Part model, mm, in its own coordinate system. Round coordinates to 2 decimals unless told otherwise and drop trailing zeros. Loops run counter-clockwise (first coordinate to the right, second up) from the corner with the lowest first, then second, coordinate; pieces in that order, holes last. Notation, with made-up numbers: M -31,42.25 L 3,42.25 A25 cw 3,64.25 Z; hole C -6.75,-31 d8. An arc over 180 degrees is marked long. Answer as CSV lines item,"result". Start each with the question number.
Item 1: Band-saw the part on B-B (x = 311.5). Give the cut face in (y, z), and give its area (3 significant figures).
Item 2: Wall check: line 1 (X direction, y = 6, z = 0.1); line 2 (Y direction, x = 303, z = 2.75); line 3 (X direction, y = 19.5, z = 2.5). Give the ranges that are in metal, low to high.
Item 3: Band-saw the part on C-C (x = 125.25). Give the cut face in (y, z), and give its area (3 significant figures).
Item 4: Drop flat-ended pins along their axis: pin 1 Ø1 at (x, y) = (124.5, 62.5) entering from -Z; pin 2 Ø1.5 at (y, z) = (8, 1) entering from +X; pin 3 Ø1.5 at (x, z) = (284, 2) entering from -Y; pin 4 Ø1 at (y, z) = (25, 0.5) entering from +X. Give the stop position or say it passes through.
Item 5: Band-saw the part on A-A (y = 8). Give the cut face in (x, z), and give its area (3 significant figures).
```python
from build123d import *

# Parameters (mm, degrees)
PAD_DEPTH = 3


with BuildPart() as part:
    # Sketch → Pad (new body)
    with BuildSketch(Plane.XY):
        with BuildLine():
            Line((0, 100.6), (0, 1))
            ThreePointArc((0, 1), (0.292893, 0.292893), (1, 0))
            Line((1, 0), (14.748, 0))
            ThreePointArc((14.748, 0), (15.455107, 0.292893), (15.748, 1))
            Line((15.748, 12.7), (15.748, 1))
            ThreePointArc((22.352, 12.7), (19.05, 16.002), (15.748, 12.7))
            Line((22.352, 12.7), (22.352, 1))
            ThreePointArc((22.352, 1), (22.644893, 0.292893), (23.352, 0))
            Line((23.352, 0), (120.948, 0))
            ThreePointArc((120.948, 0), (121.655107, 0.292893), (121.948, 1))
            Line((121.948, 12.7), (121.948, 1))
            ThreePointArc((128.552, 12.7), (125.25, 16.002), (121.948, 12.7))
            Line((128.552, 12.7), (128.552, 1))
            ThreePointArc((128.552, 1), (128.844893, 0.292893), (129.552, 0))
            Line((129.552, 0), (227.148, 0))
            ThreePointArc((227.148, 0), (227.855107, 0.292893), (228.148, 1))
            Line((228.148, 12.7), (228.148, 1))
            ThreePointArc((234.752, 12.7), (231.45, 16.002), (228.148, 12.7))
            Line((234.752, 12.7), (234.752, 1))
            ThreePointArc((234.752, 1), (235.044893, 0.292893), (235.752, 0))
            Line((235.752, 0), (249.5, 0))
            ThreePointArc((249.5, 0), (250.207107, 0.292893), (250.5, 1))
            Line((250.5, 1), (250.5, 24.9))
            ThreePointArc((251.5, 25.9), (250.792893, 25.607107), (250.5, 24.9))
            Line((251.5, 25.9), (330.9999, 25.9))
            ThreePointArc((330.9999, 25.9), (331.707007, 26.192893), (331.9999, 26.9))
            Line((331.9999, 26.9), (331.9999, 100.6))
            ThreePointArc((331.9999, 100.6), (331.707007, 101.307107), (330.9999, 101.6))
            Line((330.9999, 101.6), (1, 101.6))
            ThreePointArc((1, 101.6), (0.292893, 101.307107), (0, 100.6))
        make_face()
    extrude(amount=PAD_DEPTH)


solid = part.part
```
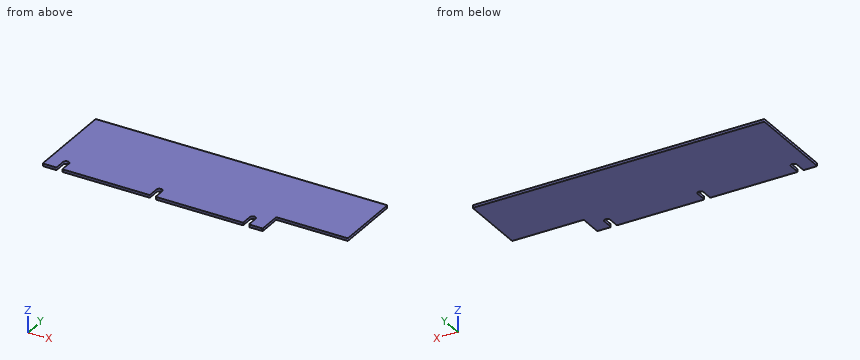
Answer block:
1,outline,"M 25.9,0 L 101.6,0 L 101.6,3 L 25.9,3 Z"
1,area,"227 mm^2"
2,line 1,"x = 0 to 15.75, 22.35 to 121.95, 128.55 to 228.15, 234.75 to 250.5"
2,line 2,"y = 25.9 to 101.6"
2,line 3,"x = 0 to 250.5"
3,outline,"M 16,0 L 101.6,0 L 101.6,3 L 16,3 Z"
3,area,"257 mm^2"
4,pin 1,"stops at z = 0"
4,pin 2,"stops at x = 250.5"
4,pin 3,"stops at y = 25.9"
4,pin 4,"stops at x = 250.7"
5,outline,"M 0,0 L 15.75,0 L 15.75,3 L 0,3 Z; M 22.35,0 L 121.95,0 L 121.95,3 L 22.35,3 Z; M 128.55,0 L 228.15,0 L 228.15,3 L 128.55,3 Z; M 234.75,0 L 250.5,0 L 250.5,3 L 234.75,3 Z"
5,area,"692 mm^2"
